Could you check a few things on this model? Use its own coordinates, in mm. A direction names the side the tool comes from. Coordinates: 2 decimals unless noted, no trailing zeros. Loops run counter-clockwise (first coordinate to the right, second up) from the corner with the lowest first, then second, coordinate; pieces in that order, holes last. Notation, with made-up numbers: M -36,-27.75 L 9,-27.75 A31 ccw 9,-3.75 Z; hole C 87.5,-13 d7. An arc over 180 degrees is marked long. Return JSON: item names as keys, results as strings. Group by question number.
from build123d import *

# Parameters (mm, degrees)
F3_T = -19.05


with BuildPart() as f2:
    # F0 (on Top) → F2 section 0
    with BuildSketch(Plane.XY, mode=Mode.PRIVATE) as f2_s0:
        Polygon((152.4, 87.988181), (-152.4, 87.988181), (0, -175.976362), align=None)
    loft([f2_s0.sketch, Vertex(0, 0, 124.4346)])

    # F3
    f3_openings = [f2.faces().sort_by_distance(p)[0] for p in [
        (0, 0, 0),
    ]]
    offset(amount=F3_T, openings=f3_openings)


solid = f2.part
(1) If I drill on L1, parallel to X at y = 4.5, z = 30; L2, parallel to X at y = 59.5, z = 7; L3, parallel to Y at x = -20, z = 67.5, over which ranges is the centre line in solid material (lowest first)? Write a range as [from, to].
(2) For faces 5 (the face through (-47.1, -24.73, 49.26)), 6 (the face through (-34.61, -18.17, 36.2)), which set-ups out of +Z, -Z, +X, -X, +Y, -Y let a thin tool reach every point of the face, with its end or its side?
(3) Will these pins go through, and if not, where does the flat tip stop? P1, Ø2, axis at x = -33.5, y = -27, coming from the -Z side; P2, Ø6, axis at x = 72.5, z = 64, coming from the -Y side; P3, Ø12, axis at x = 121.5, z = 16.5, coming from the +Y side.
(4) Imagine slicing it at A-A, the plane y = 18. Write out the boundary of the cut face in (x, z), then the cut area to 3 significant figures.
(5) We'd pull the mould along Y, two halves only. Please class faces 1 (the face through (2.134, 53.155, 49.262)), 2 (the face through (1.57, 39.06, 36.2)), 3 (the face through (33.04, -20.89, 36.2)), 4 (the face through (44.966, -28.425, 49.262)): +Y half, -Y half, draft (parallel to the pull), parting line (faces both ways), or undercut.
(6) Imagine slicing it at C-C, the plane x = 10.5. Write out the boundary of the cut face in (y, z).
(7) Imagine slicing it at B-B, the plane z = 35. Write out the boundary of the cut face in (x, y), then the cut area to 3 significant figures.
(8) Imagine slicing it at D-D, the plane z = 84.5. Write out the boundary of the cut face in (x, y), then the cut area to 3 significant figures.
Checks:
{
 "1": {"L1": "[-79.7, -52.76], [52.76, 79.7]", "L2": "[-130.24, -103.3], [103.3, 130.24]", "L3": "[-45.88, 0.79], [16.93, 40.26]"},
 "2": {"face 5": "+Z, -X, -Y", "face 6": "-Z"},
 "3": {"P1": "z = 29.9", "P2": "y = 33.4", "P3": "y = 80.56"},
 "4": {"outline": "M -111.99,0 L -85.05,0 L -31.18,65.98 L 31.18,65.98 L 85.05,0 L 111.99,0 L 31.18,98.98 L -31.18,98.98 Z", "area": "6,500 mm²"},
 "5": {"face 1": "+Y half", "face 2": "undercut", "face 3": "undercut", "face 4": "-Y half"},
 "6": {"outline": "M -157.79,0 L -111.13,0 L 6.06,82.87 L 64.66,0 L 87.99,0 L 6.06,115.86 Z"},
 "7": {"outline": "M -109.53,63.24 L 0,-126.48 L 109.53,63.24 Z; hole M -69.12,39.91 L 0,-79.82 L 69.12,39.91 Z", "area": "12,500 mm²"},
 "8": {"outline": "M -48.91,28.24 L 0,-56.48 L 48.91,28.24 Z; hole M -8.5,4.91 L 0,-9.81 L 8.5,4.91 Z", "area": "4,020 mm²"}
}
